Can you work these out from the model? Positions are in its coordinate system, mm. A direction names the side the tool comes from. Coordinates: 2 decimals unless noted, no trailing zeros. Order: outer loops, then holes, each group sorted by start corner. A loop starts at its lowest first (then second) coordinate and runs counter-clockwise, first axis right, second up. Notation, with made-up numbers: (74, 48.5) -> (124, 48.5) arc R35 ccw to (124, 80.5) -> close; hole circle Ø6 at (80.5, 42). An arc over 180 degrees is marked (long way). Answer in a Markdown table with one row per item. Add a question column.
1. If I drill on line 1 along Y through (x, z) = (0, 21.05); line 2 along Y through (x, z) = (0, 8.25); line 3 along Z through (x, y) = (-0.5, -87), over which ranges is the centre line in solid material (lowest first)? Write a range as [from, to].
2. Imagine slicing it at B-B on z = 15. Write out the boundary of the cut face in (x, y).
3. Will these pins go through, and if not, where does the flat tip stop? pin 1 (21.5 mm diameter, centred on x = 4, y = -101, fed in from +Z); pin 2 (2.5 mm diameter, centred on x = 1, y = 6, fed in from -Z); pin 3 (1.5 mm diameter, centred on x = -5, z = 20.5, fed in from -Y); pin 4 (1.5 mm diameter, centred on x = -0.5, y = -6, fed in from -Z).
4. On a 3-axis mill with a long thin cutter (end or side, diameter ignored), from which of +Z, -Z, +X, -X, +Y, -Y can I reach the whole of each face in a straight line? I mean faces 1 (the face through (-2, 7, 18)), 2 (the face through (11.4, -76.8, 7.9)), 3 (the face through (-2.38, -10.74, 17.58)). Say none if no direction works.
5. We'd pull the mould along Y, two halves only. Please class faces 4 (the face through (0, 0, 23)), 5 (the face through (0.54, 4.56, 8.87)), 6 (the face through (-22.376, -74.334, 7.944)): pulls with the +Y half, pulls with the -Y half, needs draft (parallel to the pull), parting line crosses it, or undercut.
6. Imagine slicing it at A-A on x = 0. State how many separate pieces and enclosed holes the cut face has, plus the area to 3 significant figures.
from build123d import *

# Parameters (mm, degrees)
BOSS_EXTRUDE1_DEPTH = 12
CHAMFER1_SIZE       = 4
CUT_EXTRUDE1_REACH  = 168.982
SKETCH2_R           = 1.6
CUT_EXTRUDE2_REACH  = 168.982
SKETCH3_R           = 2.5
BOSS_EXTRUDE2_START = 11
SKETCH4_R           = 11
SKETCH4_R_2         = 1.6
BOSS_EXTRUDE2_DEPTH = 11
SKETCH5_R           = 2.5
CUT_EXTRUDE3_DEPTH  = 18


with BuildPart() as part:
    # Sketch1 → Boss-Extrude1 (new body)
    with BuildSketch(Plane.XY):
        with BuildLine():
            ThreePointArc((-14.803345861, -152.420940171), (2.169116424, -164.842335865), (14.877042343, -148.083333333))
            ThreePointArc((14.877042343, -148.083333333), (11.431951297, -75.777407981), (19.625034581, -3.854609929))
            ThreePointArc((19.625034581, -3.854609929), (2.889103385, 19.790226922), (-19.907947882, 1.916666667))
            ThreePointArc((-19.907947882, 1.916666667), (-22.341608419, -75.417043737), (-14.803345861, -152.420940171))
        make_face()
    extrude(amount=BOSS_EXTRUDE1_DEPTH)

    # Chamfer1
    chamfer1_edges = [part.edges().sort_by_distance(p)[0] for p in [
        (2.889103385, 19.790226922, 0),
        (11.431951297, -75.777407981, 0),
        (2.169116424, -164.842335865, 0),
        (-22.341608419, -75.417043737, 0),
    ]]
    chamfer(chamfer1_edges, length=CHAMFER1_SIZE)

    # Sketch2 → Cut-Extrude1 (cut, up to next)
    with BuildSketch(Plane.XY.offset(12), mode=Mode.PRIVATE) as cut_extrude1_sk1:
        with Locations((0, 7)):
            Circle(SKETCH2_R)
    cut_extrude1_tool1 = extrude(cut_extrude1_sk1.sketch, amount=-CUT_EXTRUDE1_REACH, mode=Mode.PRIVATE) & part.part
    # Sketch2 → Cut-Extrude1 (cut, up to next)
    with BuildSketch(Plane.XY.offset(12), mode=Mode.PRIVATE) as cut_extrude1_sk2:
        with Locations((7, 0)):
            Circle(SKETCH2_R)
    cut_extrude1_tool2 = extrude(cut_extrude1_sk2.sketch, amount=-CUT_EXTRUDE1_REACH, mode=Mode.PRIVATE) & part.part
    # Sketch2 → Cut-Extrude1 (cut, up to next)
    with BuildSketch(Plane.XY.offset(12), mode=Mode.PRIVATE) as cut_extrude1_sk3:
        with Locations((0, -7)):
            Circle(SKETCH2_R)
    cut_extrude1_tool3 = extrude(cut_extrude1_sk3.sketch, amount=-CUT_EXTRUDE1_REACH, mode=Mode.PRIVATE) & part.part
    # Sketch2 → Cut-Extrude1 (cut, up to next)
    with BuildSketch(Plane.XY.offset(12), mode=Mode.PRIVATE) as cut_extrude1_sk4:
        with Locations((-7, 0)):
            Circle(SKETCH2_R)
    cut_extrude1_tool4 = extrude(cut_extrude1_sk4.sketch, amount=-CUT_EXTRUDE1_REACH, mode=Mode.PRIVATE) & part.part
    add(cut_extrude1_tool1.solids().sort_by_distance((0, 7, 12))[0], mode=Mode.SUBTRACT)
    add(cut_extrude1_tool2.solids().sort_by_distance((7, 0, 12))[0], mode=Mode.SUBTRACT)
    add(cut_extrude1_tool3.solids().sort_by_distance((0, -7, 12))[0], mode=Mode.SUBTRACT)
    add(cut_extrude1_tool4.solids().sort_by_distance((-7, 0, 12))[0], mode=Mode.SUBTRACT)

    # Sketch3 → Cut-Extrude2 (cut, up to next)
    with BuildSketch(Plane.XY.offset(12), mode=Mode.PRIVATE) as cut_extrude2_sk1:
        with Locations((0, -150)):
            Circle(SKETCH3_R)
    cut_extrude2_tool1 = extrude(cut_extrude2_sk1.sketch, amount=-CUT_EXTRUDE2_REACH, mode=Mode.PRIVATE) & part.part
    add(cut_extrude2_tool1.solids().sort_by_distance((0, -150, 12))[0], mode=Mode.SUBTRACT)

    # Sketch4 → Boss-Extrude2 (add)
    with BuildSketch(Plane.XY.offset(12).offset(BOSS_EXTRUDE2_START)):
        Circle(SKETCH4_R)
        with Locations((7, 0)):
            Circle(SKETCH4_R_2, mode=Mode.SUBTRACT)
        with Locations((0, -7)):
            Circle(SKETCH4_R_2, mode=Mode.SUBTRACT)
        with Locations((-7, 0)):
            Circle(SKETCH4_R_2, mode=Mode.SUBTRACT)
        with Locations((0, 7)):
            Circle(SKETCH4_R_2, mode=Mode.SUBTRACT)
    extrude(amount=-BOSS_EXTRUDE2_DEPTH)

    # Sketch5 → Cut-Extrude3 (cut)
    with BuildSketch(Plane(origin=(0, 0, 0), x_dir=(-1, 0, 0), z_dir=(0, 0, -1))):
        with Locations((0, 7)):
            Circle(SKETCH5_R)
        with Locations((7, 0)):
            Circle(SKETCH5_R)
        with Locations((0, -7)):
            Circle(SKETCH5_R)
        with Locations((-7, 0)):
            Circle(SKETCH5_R)
    extrude(amount=-CUT_EXTRUDE3_DEPTH, mode=Mode.SUBTRACT)


solid = part.part
Answers follow:
| question | item | result |
|---|---|---|
| 1 | line 1 | y = [-11, -8.6], [-5.4, 5.4], [8.6, 11] |
| 1 | line 2 | y = [-165, -152.5], [-147.5, -9.5], [-4.5, 4.5], [9.5, 20] |
| 1 | line 3 | z = [0, 12] |
| 2 | outline | circle Ø22 at (0, 0); hole circle Ø5 at (-7, 0); hole circle Ø5 at (0, -7); hole circle Ø5 at (0, 7); hole circle Ø5 at (7, 0) |
| 3 | pin 1 | stops at z = 12 |
| 3 | pin 2 | stops at z = 0 |
| 3 | pin 3 | stops at y = -10.15 |
| 3 | pin 4 | stops at z = 18 |
| 4 | face 1 | -Z |
| 4 | face 2 | +Z, -Z, +X |
| 4 | face 3 | +Z |
| 5 | face 4 | needs draft |
| 5 | face 5 | undercut |
| 5 | face 6 | parting line crosses it |
| 6 | separate pieces | 4 |
| 6 | enclosed holes | 0 |
| 6 | area | 2,170 mm² |
